```python
from build123d import *

# Parameters (mm, degrees)
SKETCH2_R           = 1.6
BOSS_EXTRUDE1_DEPTH = 4.2
CHAMFER1_SIZE       = 10


with BuildPart() as part:
    # Sketch2 → Boss-Extrude1 (new body)
    with BuildSketch(Plane(origin=(0, 0, 0), x_dir=(0, 1, 0), z_dir=(0, 0, 1))):
        with BuildLine():
            Line((0, 0), (37, 0))
            ThreePointArc((37, 0), (44.071067812, 2.928932188), (47, 10))
            Line((47, 10), (47, 47))
            ThreePointArc((47, 47), (44.071067812, 54.071067812), (37, 57))
            Line((37, 57), (0, 57))
            Line((0, 57), (0, 0))
        make_face()
        with Locations(Location((43.7, 44, 0), (0, 0, 270))):
            Circle(SKETCH2_R, mode=Mode.SUBTRACT)
        with Locations(Location((43.7, 13, 0), (0, 0, 270))):
            Circle(SKETCH2_R, mode=Mode.SUBTRACT)
        with Locations(Location((10, 45.5, 0), (0, 0, 270))):
            Circle(SKETCH2_R, mode=Mode.SUBTRACT)
        with Locations(Location((10, 11.5, 0), (0, 0, 270))):
            Circle(SKETCH2_R, mode=Mode.SUBTRACT)
        with Locations(Location((30, 45.5, 0), (0, 0, 270))):
            Circle(SKETCH2_R, mode=Mode.SUBTRACT)
        with Locations(Location((30, 11.5, 0), (0, 0, 270))):
            Circle(SKETCH2_R, mode=Mode.SUBTRACT)
    extrude(amount=BOSS_EXTRUDE1_DEPTH)

    # Chamfer1
    chamfer1_edges = [part.edges().sort_by_distance(p)[0] for p in [
        (-57, 0, 2.1),
        (0, 0, 2.1),
    ]]
    chamfer(chamfer1_edges, length=CHAMFER1_SIZE)


solid = part.part
```
Input: part model. Units: mm. Frame: model coordinates. Round coordinates to 2 decimals unless told otherwise and drop trailing zeros. Order: outer loops, then holes, each group sorted by start corner. A loop starts at its lowest first (then second) coordinate and runs counter-clockwise, first axis right, second up. Notation, with made-up numbers: (44.25, 47.25) - (80.25, 47.25) arc R20 cw to (80.25, 86.25) - close; hole circle Ø11 at (41, 79). An arc over 180 degrees is marked (long way). Answer in a Markdown table with one row per item.
Item 1: Section query C-C (x = -43). Return the cut outline in (y, z), then the cut area to 3 significant figures.
Model answer:
| item | result |
|---|---|
| outline | (0, 0) - (42.45, 0) - (42.45, 4.2) - (0, 4.2) - close; (44.95, 0) - (47, 0) - (47, 4.2) - (44.95, 4.2) - close |
| area | 187 mm² |
Item 2: Section query D-D (y = 43.7). Return the cut outline in (x, z).
Model answer:
| item | result |
|---|---|
| outline | (-54.42, 0) - (-45.6, 0) - (-45.6, 4.2) - (-54.42, 4.2) - close; (-42.4, 0) - (-14.6, 0) - (-14.6, 4.2) - (-42.4, 4.2) - close; (-11.4, 0) - (-2.58, 0) - (-2.58, 4.2) - (-11.4, 4.2) - close |
Item 3: Line query: line 1 (X direction, y = 42.5, z = 2.8); line 2 (Y direction, x = -10.5, z = 3.4); line 3 (X direction, y = 4, z = 1.9). Output: solid intervals per line, ascending.
Model answer:
| item | result |
|---|---|
| line 1 | x = -55.35 to -45.06, -42.94 to -14.06, -11.94 to -1.65 |
| line 2 | y = 0 to 8.75, 11.25 to 28.75, 31.25 to 47 |
| line 3 | x = -51 to -6 |
Item 4: Section query A-A (y = 30). Return the cut outline in (x, z).
Model answer:
| item | result |
|---|---|
| outline | (-57, 0) - (-47.1, 0) - (-47.1, 4.2) - (-57, 4.2) - close; (-43.9, 0) - (-13.1, 0) - (-13.1, 4.2) - (-43.9, 4.2) - close; (-9.9, 0) - (0, 0) - (0, 4.2) - (-9.9, 4.2) - close |
Item 5: Mould query, pull axis Y, two halves, no side actions, for faces 1 (the cylindrical face through (-2.85, 43.99, 2.07)), 2 (the flat face through (-52, 5, 2)), 3 (the cylindrical face through (-43.14, 45.05, 2.07)). Classes: released by +Y, released by -Y, zero draft, split by the parting line, or undercut.
Model answer:
| item | result |
|---|---|
| face 1 | released by +Y |
| face 2 | released by -Y |
| face 3 | undercut |
Item 6: Section query B-B (z = 3.35). Return the cut outline in (x, y), then the cut area to 3 significant figures.
Model answer:
| item | result |
|---|---|
| outline | (-57, 10) - (-47, 0) - (-10, 0) - (0, 10) - (0, 37) arc R10 ccw to (-10, 47) - (-47, 47) arc R10 ccw to (-57, 37) - close; hole circle Ø3.2 at (-45.5, 10); hole circle Ø3.2 at (-45.5, 30); hole circle Ø3.2 at (-44, 43.7); hole circle Ø3.2 at (-13, 43.7); hole circle Ø3.2 at (-11.5, 10); hole circle Ø3.2 at (-11.5, 30) |
| area | 2,490 mm² |
